from build123d import *

# Parameters (mm, degrees)
SKETCH1_W               = 2560
SKETCH1_H               = 400
BOSS_EXTRUDE1_DEPTH     = 400
SKETCH2_W               = 340
SKETCH2_H               = 360
CUT_EXTRUDE1_DEPTH      = 380
SKETCH3_W               = 100
SKETCH3_H               = 100
BOSS_EXTRUDE2_DEPTH     = 150
FILLET1_R               = 50
SKETCH4_W               = 100
SKETCH4_H               = 100
BOSS_EXTRUDE3_DEPTH     = 150
FILLET2_R               = 50
CUT_EXTRUDE2_DEPTH      = 2622.755137308
CUT_EXTRUDE2_DEPTH_BACK = 2622.755137308
SKETCH5_R               = 45


with BuildPart() as part:
    # Sketch1 → Boss-Extrude1 (new body)
    with BuildSketch(Plane.XY):
        with Locations((1280, -200)):
            Rectangle(SKETCH1_W, SKETCH1_H)
    extrude(amount=BOSS_EXTRUDE1_DEPTH)

    # Sketch2 → Cut-Extrude1 (cut)
    with BuildSketch(Plane.XY.offset(400)):
        with Locations((190, -200)):
            Rectangle(SKETCH2_W, SKETCH2_H)
        with Locations((553.333333333, -200)):
            Rectangle(SKETCH2_W, SKETCH2_H)
        with Locations((916.666666667, -200)):
            Rectangle(SKETCH2_W, SKETCH2_H)
        with Locations((1280, -200)):
            Rectangle(SKETCH2_W, SKETCH2_H)
        with Locations((1643.333333333, -200)):
            Rectangle(SKETCH2_W, SKETCH2_H)
        with Locations((2006.666666667, -200)):
            Rectangle(SKETCH2_W, SKETCH2_H)
        with Locations((2370, -200)):
            Rectangle(SKETCH2_W, SKETCH2_H)
    extrude(amount=-CUT_EXTRUDE1_DEPTH, mode=Mode.SUBTRACT)

    # Sketch3 → Boss-Extrude2 (add)
    with BuildSketch(Plane(origin=(0, 0, 0), x_dir=(1, 0, 0), z_dir=(0, 1, 0))):
        with Locations((50, -200)):
            Rectangle(SKETCH3_W, SKETCH3_H)
    extrude(amount=BOSS_EXTRUDE2_DEPTH)

    # Fillet1
    fillet1_edges = [part.edges().sort_by_distance(p)[0] for p in [
        (50, 150, 150),
        (50, 150, 250),
    ]]
    fillet(fillet1_edges, radius=FILLET1_R - 0.0001)  # a hair under: the kernel refuses the full size

    # Sketch4 → Boss-Extrude3 (add)
    with BuildSketch(Plane(origin=(0, 0, 0), x_dir=(1, 0, 0), z_dir=(0, 1, 0))):
        with Locations((2510, -200)):
            Rectangle(SKETCH4_W, SKETCH4_H)
    extrude(amount=BOSS_EXTRUDE3_DEPTH)

    # Fillet2
    fillet2_edges = [part.edges().sort_by_distance(p)[0] for p in [
        (2510, 150, 150),
        (2510, 150, 250),
    ]]
    fillet(fillet2_edges, radius=FILLET2_R - 0.0001)  # a hair under: the kernel refuses the full size

    # Sketch5 → Cut-Extrude2 (cut, two sides: drawn at the far end of the back side and taken through both)
    with BuildSketch(Plane(origin=(2560, 0, 0), x_dir=(0, 0, -1), z_dir=(1, 0, 0)).offset(-CUT_EXTRUDE2_DEPTH_BACK)):
        with Locations((-200, 100)):
            Circle(SKETCH5_R)
    extrude(amount=CUT_EXTRUDE2_DEPTH + CUT_EXTRUDE2_DEPTH_BACK, mode=Mode.SUBTRACT)


solid = part.part
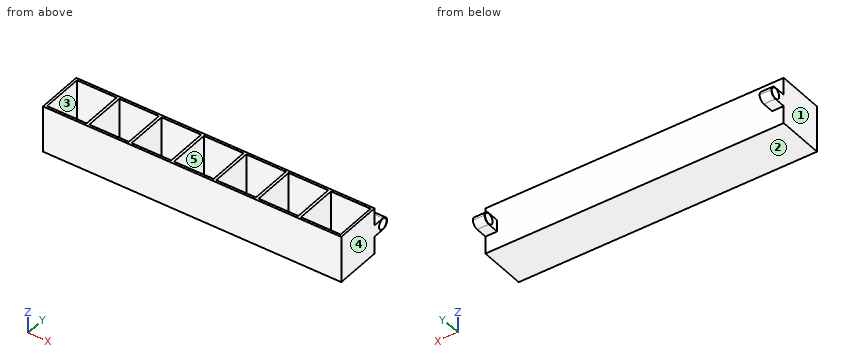
CAD build for the part. Positions are in the model's coordinates, mm. Face numbers are marked on the shaded views. A direction names the side the tool comes from. Coordinates: 2 decimals unless noted, no trailing zeros. Write each loop counter-clockwise with the first axis right and the second up, starting at its lowest first coordinate (ties: lowest second). Pieces come first, ordered by that corner, then holes. Notation, with made-up numbers: M -8,-38.5 L 2,-38.5 A13 ccw 2,-16.5 Z; hole C 57.25,-24.5 d6. An arc over 180 degrees is marked long. Return JSON: item names as keys, results as strings.
Item 1: Two-plate mould, pull along X, no slides. Class the marked faces 1, 2 and 3: +X half, -X half, draft (parallel to the pull), parting line (faces both ways), or undercut.
Findings below:
{"face 1": "-X half", "face 2": "draft", "face 3": "undercut"}
Item 2: Probe line 1 (Y direction, x = 2165, z = 125); line 2 (Y direction, x = 2518.5, z = 200); line 3 (Z direction, x = 1080.5, y = -294). List the from-to ranges inside material, lowest first. Write a range as from..to.
Findings below:
{"line 1": "y = -400..-380, -20..0", "line 2": "y = -400..-380, -20..55, 145..150", "line 3": "z = 0..20"}
Item 3: Which spindle directions (+Z, -Z, +X, -X, +Y, -Y) get a long thin tool onto all of the face, cutting with end or side? Do the marked faces 4 and 5. Say none if no direction does.
Findings below:
{"face 4": "+Z, -Z, +X, +Y, -Y", "face 5": "+Z"}
Item 4: Slice it at B-B, the plane z = 304.5. State how many separate pieces and enclosed holes the cut face has, and give its area (3 significant figures).
Findings below:
{"separate pieces": "1", "enclosed holes": "7", "area": "167,000 mm2"}
Item 5: Slice it at C-C, the plane x = 1603. Write the cut outline in (y, z), and give its area (3 significant figures).
Findings below:
{"outline": "M -400,0 L 0,0 L 0,400 L -20,400 L -20,20 L -380,20 L -380,400 L -400,400 Z", "area": "23,200 mm2"}
Item 6: Drop a flat-ended pin along its axis: pin 1 Ø8 at (x, z) = (1832.5, 316.5) entering from +Y. Give the stop position or say it passes through.
Findings below:
{"pin 1": "stops at y = 0"}
Item 7: Slice it at A-A, the plane y = 78. Write the cut outline in (x, z).
Findings below:
{"outline": "M 0,150 L 100,150 L 100,160.74 L 0,160.74 Z; M 0,239.26 L 100,239.26 L 100,250 L 0,250 Z; M 2460,150 L 2560,150 L 2560,160.74 L 2460,160.74 Z; M 2460,239.26 L 2560,239.26 L 2560,250 L 2460,250 Z"}
